```python
from build123d import *

# Parameters (mm, degrees)
F1_DEPTH       = 63.5
F3_DEPTH       = 15.748
F5_DEPTH       = 4.826
F7_DEPTH       = 55.118
F9_D           = 12.7
F9_CBORE_D     = 19.05
F9_CBORE_DEPTH = 9.652


with BuildPart() as f1:
    # F0 (on Front) → F1 (new body)
    with BuildSketch(Plane.XZ):
        Polygon((-3.422344, 11.084872), (-3.422344, 26.832872), (-54.222344, 26.832872), (-54.222344, -7.965128), (-22.472344, -7.965128), (-22.472344, -12.791128), (-3.422344, -12.791128), (-3.422344, -7.965128), (28.327656, -7.965128), (28.327656, 11.084872), align=None)
    extrude(amount=F1_DEPTH)

    # F2 (on face) → F3 (cut)
    with BuildSketch(Plane.XY.offset(26.832872)):
        Polygon((-3.422344, -10.526553), (-47.872344, -63.5), (-3.422344, -63.5), align=None)
    extrude(amount=-F3_DEPTH, mode=Mode.SUBTRACT)

    # F4 (on face) → F5 (cut)
    with BuildSketch(Plane.XY.offset(11.084872)):
        Polygon((2.927656, -63.5), (28.327656, -63.5), (28.327656, -33.229459), align=None)
    extrude(amount=-F5_DEPTH, mode=Mode.SUBTRACT)

    # F6 (on face) → F7 (cut)
    with BuildSketch(Plane.YZ.offset(-3.422344)):
        Polygon((0, 13.048057), (0, 26.832872), (-23.876, 26.832872), align=None)
    extrude(amount=-F7_DEPTH, mode=Mode.SUBTRACT)

    # F9 (through all)
    with Locations(Plane.XY.offset(11.084872)):
        with Locations((-12.820344, -44.45)):
            CounterBoreHole(F9_D / 2, F9_CBORE_D / 2, F9_CBORE_DEPTH)


solid = f1.part
```
Build history of the part. All positions in model axes, mm. A direction names the side the tool comes from. Coordinates: 2 decimals unless noted, no trailing zeros. Order: outer loops, then holes, each group sorted by start corner. A loop starts at its lowest first (then second) coordinate and runs counter-clockwise, first axis right, second up.
Item 1: Drill centre lines: L1, parallel to Y at x = -13, z = -6; L2, parallel to Y at x = -10, z = 1.5; L3, parallel to X at y = -44, z = -7. Where is each one in solid material? Low to high.
Filled in:
L1: y = -63.5 to -50.8, -38.1 to 0
L2: y = -63.5 to -53.55, -35.35 to 0
L3: x = -54.22 to -19.15, -6.49 to 28.33
Item 2: Mould opens along Y. For faces 1 (the flat face through (-54.222, -31, 10)), 2 (the flat face through (-28.47, -12.11, 20.04)), 3 (the cylindrical face through (-11.994, -38.154, -5.779)) say: released by +Y, released by -Y, zero draft, split by the parting line, or undercut.
Filled in:
face 1: zero draft
face 2: released by +Y
face 3: undercut
Item 3: Tool access for faces 4 (the flat face through (-3.422, -6, 14)), 5 (the flat face through (21, -55, 6.259)), 6 (the flat face through (-39, -31, -7.965)): list every direction of +Z, -Z, +X, -X, +Y, -Y with a clear straight run to the whole face (end or side of a thin tool).
Filled in:
face 4: +Z, +X, +Y, -Y
face 5: +Z, +X, -Y
face 6: -Z, -X, +Y, -Y
Item 4: Saw through at B-B on y = -44.45. List the corners of the cut face in (x, z).
Filled in:
outline: (-54.22, -7.97) - (-22.47, -7.97) - (-22.47, -12.79) - (-19.17, -12.79) - (-19.17, 1.43) - (-22.35, 1.43) - (-22.35, 11.08) - (-31.89, 11.08) - (-31.89, 26.83) - (-54.22, 26.83) - close; (-6.47, -12.79) - (-3.42, -12.79) - (-3.42, -7.97) - (28.33, -7.97) - (28.33, 6.26) - (18.91, 6.26) - (18.91, 11.08) - (-3.3, 11.08) - (-3.3, 1.43) - (-6.47, 1.43) - close
Item 5: Saw through at A-A on z = -1. List the corners of the cut face in (x, y), then the cut area to 3 significant figures.
Filled in:
outline: (-54.22, -63.5) - (28.33, -63.5) - (28.33, 0) - (-54.22, 0) - close; hole circle Ø12.7 at (-12.82, -44.45)
area: 5,120 mm2
Item 6: Drop flat-ended pins along their axis: pin 1 Ø19 at (x, y) = (-14, -43.5) entering from +Z; pin 2 Ø1.5 at (x, y) = (19.5, -18.5) entering from -Z; pin 3 Ø4 at (y, z) = (-18, -11) entering from +X. Give the stop position or say it passes through.
Filled in:
pin 1: stops at z = 11.08
pin 2: stops at z = -7.97
pin 3: stops at x = -3.42
Item 7: Saw through at D-D on y = -26.5. List the corners of the cut face in (x, z), then the cut area to 3 significant figures.
Filled in:
outline: (-54.22, -7.97) - (-22.47, -7.97) - (-22.47, -12.79) - (-3.42, -12.79) - (-3.42, -7.97) - (28.33, -7.97) - (28.33, 11.08) - (-16.83, 11.08) - (-16.83, 26.83) - (-54.22, 26.83) - close
area: 2,250 mm2
Item 8: Saw through at C-C on x = -39.5. List the corners of the cut face in (y, z).
Filled in:
outline: (-63.5, -7.97) - (0, -7.97) - (0, 13.05) - (-23.88, 26.83) - (-53.52, 26.83) - (-53.52, 11.08) - (-63.5, 11.08) - close
